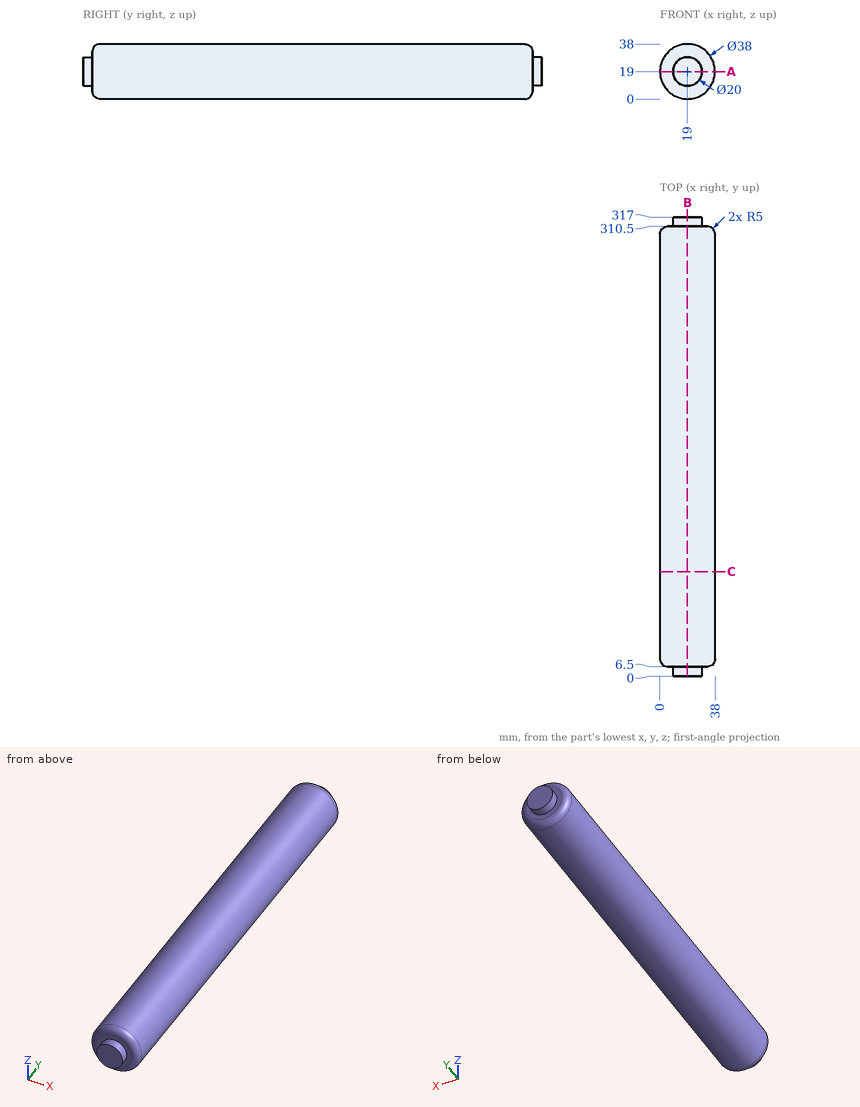
The figure shows three views and two pictorial views of one solid part (mm, origin at its lowest corner). Answer the questions. Round coordinates to 2 decimals unless told otherwise and drop trailing zeros. Write each loop counter-clockwise with the first axis right and the second up, starting at its lowest first coordinate (ties: lowest second). Pieces come first, ordered by that corner, then holes. Notation, with made-up numbers: M 81,18.25 L 113,18.25 A7 cw 113,24.25 Z; hole C 83,-18.75 d1. An arc over 180 degrees is marked long. Use a Markdown table: item, result.
1) Straight lines are drawn through the part: line 1 along Z through (x, y) = (18, 96.5); line 2 along X through (y, z) = (245, 19.5); line 3 along Y through (x, z) = (33, 18). For each, find the intervals that lie inside material, in ascending order. Write a range as [from, to].
Answers follow:
| item | result |
|---|---|
| line 1 | z = [0.03, 37.97] |
| line 2 | x = [0.01, 37.99] |
| line 3 | y = [6.5, 310.5] |
2) The part is cut by section B-B (x = 19). Write down the section's boundary in (y, z), plus the area to 3 significant figures.
Answers follow:
| item | result |
|---|---|
| outline | M 0,9 L 6.5,9 L 6.5,5 A5 ccw 11.5,0 L 305.5,0 A5 ccw 310.5,5 L 310.5,9 L 317,9 L 317,29 L 310.5,29 L 310.5,33 A5 ccw 305.5,38 L 11.5,38 A5 ccw 6.5,33 L 6.5,29 L 0,29 Z |
| area | 11,800 mm2 |
3) Flat-ended cylindrical pins translate along their axes: pin 1 (12 mm diameter, centred on x = 12, y = 226, fed in from -Z); pin 2 (4 mm diameter, centred on x = 9, y = 141, fed in from +Z); pin 3 (1 mm diameter, centred on x = 7, y = 135.5, fed in from +Z). Find the tip coordinate at first contact, or state that the pin passes through.
Answers follow:
| item | result |
|---|---|
| pin 1 | stops at z = 0.03 |
| pin 2 | stops at z = 36.23 |
| pin 3 | stops at z = 34.12 |
4) The part is cut by section A-A (z = 19). Write down the section's boundary in (x, y), plus the area to 3 significant figures.
Answers follow:
| item | result |
|---|---|
| outline | M 0,11.5 A5 ccw 5,6.5 L 9,6.5 L 9,0 L 29,0 L 29,6.5 L 33,6.5 A5 ccw 38,11.5 L 38,305.5 A5 ccw 33,310.5 L 29,310.5 L 29,317 L 9,317 L 9,310.5 L 5,310.5 A5 ccw 0,305.5 Z |
| area | 11,800 mm2 |
5) The part is cut by section C-C (y = 72). Write down the section's boundary in (x, z).
Answers follow:
| item | result |
|---|---|
| outline | C 19,19 d38 |
